Could you check a few things on this drawing? It's one solid part, dimensions in mm from its lowest x, y, z. Round coordinates to 2 decimals unless told otherwise and drop trailing zeros. Write each loop counter-clockwise with the first axis right and the second up, starting at its lowest first coordinate (ties: lowest second). Pieces come first, ordered by that corner, then holes. Notation, with made-up numbers: (39.5, 45) -> (54.5, 45) arc R13 ccw to (54.5, 60) -> close; hole circle Ø1 at (-22, 68.25). An arc over 180 degrees is marked (long way). Answer as CSV lines item,"result".
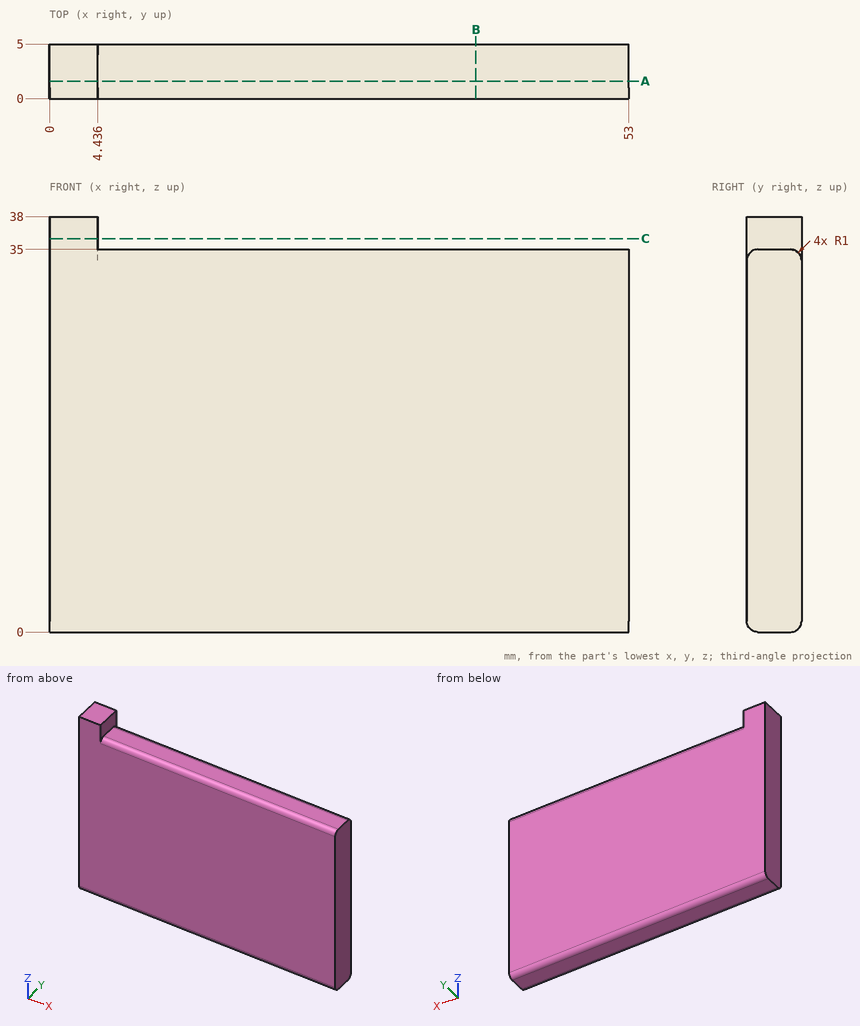
1. Suppose I cut it at C-C on z = 36. Please give me the cut outline in (x, y).
Numbers:
outline,"(0, 0) -> (4.44, 0) -> (4.44, 5) -> (0, 5) -> close"
2. Suppose I cut it at A-A on y = 1.6. Please give me the cut outline in (x, z).
Numbers:
outline,"(0, 0) -> (53, 0) -> (53, 35) -> (4.44, 35) -> (4.44, 38) -> (0, 38) -> close"
3. If I drill on line 1 (Z direction, x = 29, y = 1.2); line 2 (X direction, y = 3.55, z = 35.5); line 3 (Z direction, x = 47, y = 4.6), over which ranges is the centre line in solid material (lowest first)?
Numbers:
line 1,"z = 0 to 35"
line 2,"x = 0 to 4.44"
line 3,"z = 0.2 to 34.8"
4. Suppose I cut it at B-B on x = 39. Please give me the cut outline in (y, z).
Numbers:
outline,"(0, 1) arc R1 ccw to (1, 0) -> (4, 0) arc R1 ccw to (5, 1) -> (5, 34) arc R1 ccw to (4, 35) -> (1, 35) arc R1 ccw to (0, 34) -> close"
5. For pin 1 Ø1 at (y, z) = (1.5, 23.5) entering from -X; pin 2 Ø3 at (x, y) = (12.5, 1.5) entering from +Z, each with a flat end and sliding along its axis, tell me the tip position at first contact or that it passes through.
Numbers:
pin 1,"stops at x = 0"
pin 2,"stops at z = 35"
